```python
from build123d import *

# Parameters (mm, degrees)
F0_W           = 50
F0_H           = 65
F1_DEPTH       = 6
F2_W           = 15
F2_H           = 10
F3_DEPTH       = 41
F5_D           = 3.2
F5_CBORE_D     = 6
F5_CBORE_DEPTH = 3.5
F7_D           = 2.2
F9_DEPTH       = 15


with BuildPart() as f1:
    # F0 (on Top) → F1 (new body)
    with BuildSketch(Plane.XY):
        with Locations((25, 32.5)):
            Rectangle(F0_W, F0_H)
    extrude(amount=F1_DEPTH)

    # F2 (on face) → F3 (join)
    with BuildSketch(Plane.XY.offset(6)):
        with Locations((25, 55)):
            Rectangle(F2_W, F2_H)
    extrude(amount=F3_DEPTH)

    # F5 (through all)
    with Locations(Plane.XY.offset(6)):
        with Locations((12, 55), (38, 55), (25, 32.48334)):
            CounterBoreHole(F5_D / 2, F5_CBORE_D / 2, F5_CBORE_DEPTH)

    # F7 (through all)
    with Locations(Plane.XY.offset(6)):
        with Locations((11, 25), (39, 25), (39, 5), (11, 5), (44.5, 35)):
            Hole(F7_D / 2)

    # F8 (on face) → F9 (cut, through all)
    with BuildSketch(Plane.YZ.offset(32.5)):
        Polygon((60, 47), (50, 47), (60, 41.226497), align=None)
    extrude(amount=-F9_DEPTH, mode=Mode.SUBTRACT)


solid = f1.part
```
Geometry check sheet. Reference: the model listing, model coordinates, mm. A direction names the side the tool comes from. Coordinates: 2 decimals unless noted, no trailing zeros. Order: outer loops, then holes, each group sorted by start corner. A loop starts at its lowest first (then second) coordinate and runs counter-clockwise, first axis right, second up.
Item 1: Section check C-C (x = 19.5). Enter the section's corners in (y, z).
Item 2: Tool access check on faces 1 (the flat face through (25, 50, 26)), 2 (the flat face through (13.3, 53.7, 2.5)), 3 (the cylindrical face through (37.95, 5.33, 2.96)), 4 (the flat face through (17.5, 55, 26)), 5 (the flat face through (32.5, 55, 26)). Record the directions out of +Z, -Z, +X, -X, +Y, -Y that give a thin tool (end or side, any length) a straight path to the whole face; none if there is none.
Item 3: Section check B-B (y = 5). Enter the section's corners in (x, z), plus the area to 3 significant figures.
Item 4: Scan lines: line 1 along Y through (x, z) = (38, 4.05); line 2 along Y through (x, z) = (39, 1); line 3 along Y through (x, z) = (25, 4.85). Record each from-to range of solid material in increasing order.
Item 5: Depth check by flat-ended pin: pin 1 (3 mm diameter, centred on x = 20, y = 20.5, fed in from +Z); pin 2 (3 mm diameter, centred on y = 55, z = 24, fed in from -X); pin 3 (1.9 mm diameter, centred on x = 12, y = 55, fed in from +Z); pin 4 (10 mm diameter, centred on x = 19, z = 29, fed in from -Y). Enter the tip coordinate at first touch or a pass-through.
Item 6: Section check A-A (x = 44.5). Enter the section's corners in (y, z).
Item 7: Section check D-D (x = 25). Enter the section's corners in (y, z), plus the area to 3 significant figures.
Check sheet entries:
1. outline: (0, 0) - (65, 0) - (65, 6) - (60, 6) - (60, 41.23) - (50, 47) - (50, 6) - (0, 6) - close
2. face 1: +Z, +X, -X, -Y
2. face 2: +Z
2. face 3: +Z, -Z
2. face 4: +Z, -X, +Y, -Y
2. face 5: +Z, +X, +Y, -Y
3. outline: (0, 0) - (9.9, 0) - (9.9, 6) - (0, 6) - close; (12.1, 0) - (37.9, 0) - (37.9, 6) - (12.1, 6) - close; (40.1, 0) - (50, 0) - (50, 6) - (40.1, 6) - close
3. area: 274 mm2
4. line 1: y = 0 to 4.54, 5.46 to 24.54, 25.46 to 52, 58 to 65
4. line 2: y = 0 to 3.9, 6.1 to 23.9, 26.1 to 53.75, 56.25 to 65
4. line 3: y = 0 to 29.48, 35.48 to 65
5. pin 1: stops at z = 6
5. pin 2: stops at x = 17.5
5. pin 3: passes through
5. pin 4: stops at y = 50
6. outline: (0, 0) - (33.9, 0) - (33.9, 6) - (0, 6) - close; (36.1, 0) - (65, 0) - (65, 6) - (36.1, 6) - close
7. outline: (0, 0) - (30.88, 0) - (30.88, 2.5) - (29.48, 2.5) - (29.48, 6) - (0, 6) - close; (34.08, 0) - (65, 0) - (65, 6) - (60, 6) - (60, 41.23) - (50, 47) - (50, 6) - (35.48, 6) - (35.48, 2.5) - (34.08, 2.5) - close
7. area: 742 mm2
